Model file for the job. Use its own axes, mm. A direction names the side the tool comes from. Coordinates: 2 decimals unless noted, no trailing zeros. Order: outer loops, then holes, each group sorted by start corner. A loop starts at its lowest first (then second) coordinate and runs counter-clockwise, first axis right, second up. Notation, with made-up numbers: M -25,35.25 L 14,35.25 A29 ccw 14,64.25 Z; hole C -4.5,41.25 d10. An arc over 180 degrees is marked long. Return JSON: item names as keys, results as strings.
```python
from build123d import *

# Parameters (mm, degrees)
BOSS_EXTRUDE1_DEPTH      = 15
BOSS_EXTRUDE1_DEPTH_BACK = 3
SKETCH1_R                = 10.175
SKETCH1_R_2              = 3.2
SKETCH1_3_R              = 19
SKETCH1_3_R_2            = 10.175
BOSS_EXTRUDE2_DEPTH      = 3
SKETCH2_R                = 1.25
CUT_EXTRUDE1_DEPTH       = 15
SKETCH4_R                = 4.5
BOSS_EXTRUDE3_DEPTH      = 10
SKETCH1_7_R              = 3.2
CUT_EXTRUDE2_DEPTH       = 13
SKETCH3_R                = 1.5
CUT_EXTRUDE3_DEPTH       = 10


with BuildPart() as part:
    # Sketch1 → Boss-Extrude1 (new, two sides: drawn at the far end of the back side and taken through both)
    with BuildSketch(Plane(origin=(0, 0, 0), x_dir=(1, 0, 0), z_dir=(0, 1, 0)).offset(-BOSS_EXTRUDE1_DEPTH_BACK)):
        with Locations(Location((0, 0, 0), (0, 0, 270))):
            Circle(SKETCH1_R)
        with Locations(Location((0, 0, 0), (0, 0, 270))):
            Circle(SKETCH1_R_2, mode=Mode.SUBTRACT)
    extrude(amount=BOSS_EXTRUDE1_DEPTH + BOSS_EXTRUDE1_DEPTH_BACK)

    # Sketch2 → Cut-Extrude1 (cut)
    with BuildSketch(Plane(origin=(0, 0, 0), x_dir=(0, 0, -1), z_dir=(1, 0, 0))):
        with Locations((0, 6.702870317)):
            Circle(SKETCH2_R)
    extrude(amount=-CUT_EXTRUDE1_DEPTH, mode=Mode.SUBTRACT)


with BuildPart() as body_2:
    # Sketch1_3 → Boss-Extrude2 (new body)
    with BuildSketch(Plane(origin=(0, 0, 0), x_dir=(1, 0, 0), z_dir=(0, 1, 0))):
        with Locations(Location((0, 0, 0), (0, 0, 270))):
            Circle(SKETCH1_3_R)
        with Locations(Location((0, 0, 0), (0, 0, 270))):
            Circle(SKETCH1_3_R_2, mode=Mode.SUBTRACT)
    extrude(amount=-BOSS_EXTRUDE2_DEPTH)


    add(part.part)  # Boss-Extrude3 merges part
    # Sketch4 → Boss-Extrude3 (add)
    with BuildSketch(Plane.XZ.offset(3)):
        with Locations(Location((0, 0, 0), (0, 0, 90))):
            Circle(SKETCH4_R)
    extrude(amount=BOSS_EXTRUDE3_DEPTH)

    # Sketch1_7 → Cut-Extrude2 (cut)
    with BuildSketch(Plane(origin=(0, 0, 0), x_dir=(1, 0, 0), z_dir=(0, 1, 0))):
        with Locations(Location((0, 0, 0), (0, 0, 270))):
            Circle(SKETCH1_7_R)
    extrude(amount=-CUT_EXTRUDE2_DEPTH, mode=Mode.SUBTRACT)

    # Sketch3 → Cut-Extrude3 (cut)
    with BuildSketch(Plane.XZ.offset(3)):
        with Locations(Location((0, 16.112537947, 0), (0, 0, 270))):
            Circle(SKETCH3_R)
        with Locations(Location((12.597289429, 10.046003092, 0), (0, 0, 270))):
            Circle(SKETCH3_R)
        with Locations(Location((15.70856298, -3.585376992, 0), (0, 0, 270))):
            Circle(SKETCH3_R)
        with Locations(Location((6.990968211, -14.516895073, 0), (0, 0, 270))):
            Circle(SKETCH3_R)
        with Locations(Location((-6.990968211, -14.516895073, 0), (0, 0, 270))):
            Circle(SKETCH3_R)
        with Locations(Location((-15.70856298, -3.585376992, 0), (0, 0, 270))):
            Circle(SKETCH3_R)
        with Locations(Location((-12.597289429, 10.046003092, 0), (0, 0, 270))):
            Circle(SKETCH3_R)
    extrude(amount=-CUT_EXTRUDE3_DEPTH, mode=Mode.SUBTRACT)


solid = body_2.part
```
Item 1: Wall check: line 1 (Y direction, x = -10, z = -10); line 2 (Z direction, x = -6.5, y = -1.25); line 3 (X direction, y = 7, z = 0) (3 decimals). Give the ranges that are in metal, low to high.
Check result:
{"line 1": "y = -3 to 0", "line 2": "z = -17.85 to -15.93, -13.1 to 17.85", "line 3": "x = 3.2 to 10.175"}
Item 2: Saw through at A-A (x = 0). Write the cut outline in (y, z) (3 decimals).
Check result:
{"outline": "M -13,-4.5 L -3,-4.5 L -3,-19 L 0,-19 L 0,-10.175 L 15,-10.175 L 15,-3.2 L -13,-3.2 Z; M -13,3.2 L 15,3.2 L 15,10.175 L 0,10.175 L 0,14.613 L -3,14.613 L -3,4.5 L -13,4.5 Z; M -3,17.613 L 0,17.613 L 0,19 L -3,19 Z"}
Item 3: 3-axis set-ups, long thin cutter, end or side, ignore diameter. For faces 5 (the flat face through (-8, 0, 8)), 6 (the cylindrical face through (-6.511, 5.483, 0.271)), 7 (the cylindrical face through (-1.352, -7.93, 4.292)), 8 (the cylindrical face through (2.7, 1.2, 1.72)): which of +Z, -Z, +X, -X, +Y, -Y reach the whole face in a straight line?
Check result:
{"face 5": "+Y", "face 6": "-X", "face 7": "-Y", "face 8": "+Y, -Y"}
Item 4: Pull direction X, two halves, no side cores. Call faces 1 (the cylindrical face through (16.973, -1.521, -4.392)), 2 (the cylindrical face through (3.056, 7.395, 9.705)), 3 (the cylindrical face through (-15.258, -1.521, -5.016)), 4 (the flat face through (-4, -3, 4)): +X half, -X half, draft (parallel to the pull), parting line (faces both ways), or undercut.
Check result:
{"face 1": "undercut", "face 2": "parting line", "face 3": "undercut", "face 4": "draft"}
Item 5: Saw through at D-D (y = 9.5). Write the cut outline in (x, z) (3 decimals).
Check result:
{"outline": "C 0,0 d20.35; hole C 0,0 d6.4"}
Item 6: Drop flat-ended pins along their axis: pin 1 Ø2 at (y, z) = (6.7, 0) entering from +X (3 decimals); pin 2 Ø3 at (x, y) = (-5.5, -9.5) entering from -Z; pin 3 Ø6 at (x, z) = (-9, 10) entering from -Y. Give the stop position or say it passes through.
Check result:
{"pin 1": "stops at x = 10.175", "pin 2": "stops at z = -2.06", "pin 3": "stops at y = -3"}
Item 7: Saw through at B-B (z = 0). Write the cut outline in (x, y) (3 decimals).
Check result:
{"outline": "M -19,-3 L -4.5,-3 L -4.5,-13 L -3.2,-13 L -3.2,5.453 L -10.175,5.453 L -10.175,0 L -19,0 Z; M -10.175,7.953 L -3.2,7.953 L -3.2,15 L -10.175,15 Z; M 3.2,-13 L 4.5,-13 L 4.5,-3 L 19,-3 L 19,0 L 10.175,0 L 10.175,15 L 3.2,15 Z"}
Item 8: Saw through at C-C (x = 16.5). Write the cut outline in (y, z), and give its area (3 significant figures).
Check result:
{"outline": "M -3,-9.42 L 0,-9.42 L 0,-4.86 L -3,-4.86 Z; M -3,-2.31 L 0,-2.31 L 0,9.42 L -3,9.42 Z", "area": "48.9 mm2"}
